Design review of the part built by this model. Coordinates are the model's own, in mm. A direction names the side the tool comes from. Coordinates: 2 decimals unless noted, no trailing zeros. Write each loop counter-clockwise with the first axis right and the second up, starting at its lowest first coordinate (ties: lowest second). Pieces come first, ordered by that corner, then holes. Notation, with made-up numbers: (-16.5, 12) - (36.5, 12) arc R26 ccw to (36.5, 37) - close; hole circle Ø1 at (-24, -22.75). An arc over 180 degrees is marked (long way). One line per item, written item: value.
from build123d import *

# Parameters (mm, degrees)
F0_R      = 38.1
F1_DEPTH  = 25.4
F2_W      = 25.4
F2_H      = 25.4
F3_DEPTH  = 25.4
F4_R      = 25.4
F5_DEPTH  = 25.4
F6_W      = 25.4
F6_H      = 25.4
F7_DEPTH  = 166
F8_W      = 25.4
F8_H      = 25.4
F9_DEPTH  = 76.201
F10_R     = 12.7
F11_DEPTH = 38.101
F12_DEPTH = 50.8
F13_W     = 25.4
F13_H     = 25.4
F14_DEPTH = 38.1010001
F15_W     = 25.4
F15_H     = 25.4
F16_DEPTH = 50.8010001


# Not quite as in the source:
# - an extrude ends at something that could not be found from the text; its depth is read off the source's solid


with BuildPart() as f1:
    # F0 (on Top) → F1 (new body)
    with BuildSketch(Plane.XY):
        Circle(F0_R)
    extrude(amount=F1_DEPTH)

    # F2 (on face) → F3 (join)
    with BuildSketch(Plane.XY.offset(25.4)):
        Rectangle(F2_W, F2_H)
    extrude(amount=F3_DEPTH)

    # F4 (on face) → F5 (join)
    with BuildSketch(Plane(origin=(0, 0, 0), x_dir=(1, 0, 0), z_dir=(0, 0, -1))):
        Circle(F4_R)
    extrude(amount=F5_DEPTH)

    # F6 (on face) → F7 (cut, through all)
    with BuildSketch(Plane(origin=(0, 0, -25.4), x_dir=(1, 0, 0), z_dir=(0, 0, -1))):
        Rectangle(F6_W, F6_H)
    extrude(amount=F7_DEPTH, mode=Mode.SUBTRACT)

    # F8 (on face) → F9 (cut, through all)
    with BuildSketch(Plane(origin=(0, 0, -25.4), x_dir=(1, 0, 0), z_dir=(0, 0, -1))):
        Rectangle(F8_W, F8_H)
    extrude(amount=-F9_DEPTH, mode=Mode.SUBTRACT)

    # F10 (on Front) → F11 (cut, through all)
    with BuildSketch(Plane.XZ):
        Circle(F10_R)
    extrude(amount=-F11_DEPTH, mode=Mode.SUBTRACT)

    # F10 (on Front) → F12 (cut)
    with BuildSketch(Plane.XZ):
        Circle(F10_R)
    extrude(amount=F12_DEPTH, mode=Mode.SUBTRACT)

    # F13 (on Right) → F14 (cut, through all)
    with BuildSketch(Plane.YZ):
        Rectangle(F13_W, F13_H)
    extrude(amount=-F14_DEPTH, mode=Mode.SUBTRACT)

    # F15 (on face) → F16 (cut, through all)
    with BuildSketch(Plane.YZ.offset(-12.7)):
        Rectangle(F15_W, F15_H)
    extrude(amount=F16_DEPTH, mode=Mode.SUBTRACT)


solid = f1.part
1. Consider section D-D, the plane z = 21.5. Write out the cut boundary in (x, y).
Answer block:
outline: circle Ø76.2 at (0, 0); hole (-12.7, -12.7) - (12.7, -12.7) - (12.7, 12.7) - (-12.7, 12.7) - close
2. Consider section C-C, the plane z = 8. Write out the cut boundary in (x, y).
Answer block:
outline: (-35.92, -12.7) arc R38.1 ccw to (-9.86, -36.8) - (-9.86, -12.7) - close; (-35.92, 12.7) - (-9.86, 12.7) - (-9.86, 36.8) arc R38.1 ccw to start; (9.86, -36.8) arc R38.1 ccw to (35.92, -12.7) - (9.86, -12.7) - close; (9.86, 12.7) - (35.92, 12.7) arc R38.1 ccw to (9.86, 36.8) - close
3. For faces 1 (the face through (-18.72, -17.17, -15.34)), 2 (the face through (-19, 0, -12.7)), 3 (the face through (-12.7, 0, -19)), list the 3-axis set-ups (+Z, -Z, +X, -X, +Y, -Y) from which the entire face can be reached by the end or side of a thin tool; tool diameter is ignored.
Answer block:
face 1: -Z
face 2: +X, -X
face 3: +Z, -Z
4. Mouldability with a two-part tool opening along Y and no side actions: class faces 4 (the face through (-25, 0, 12.7)), 5 (the face through (0, 17, -25.4)), 6 (the face through (17.58, -33.8, 15.34)) as released by +Y, released by -Y, zero draft, split by the parting line, or undercut.
Answer block:
face 4: undercut
face 5: zero draft
face 6: split by the parting line
5. Wall thickness on line 1 along Z through (x, y) = (0, -18.25); line 2 along Y through (x, z) = (-25, 6.5); line 3 along Y through (x, z) = (13.5, 5): over which ranges is each line inside the solid? List them lowest first.
Answer block:
line 1: z = -25.4 to -12.7, 12.7 to 25.4
line 2: y = -28.75 to -12.7, 12.7 to 28.75
line 3: y = -35.63 to -12.7, 12.7 to 35.63
6. Insertion check: pin 1 Ø8 at (x, z) = (-9, 5) entering from -Y; pin 2 Ø10 at (y, z) = (5.5, -16.5) entering from -X; pin 3 Ø11.5 at (x, y) = (-22, -22.5) entering from -Z. Each pin has a flat end and moves straight along its axis. Give the tip position at first contact, or say it passes through.
Answer block:
pin 1: stops at y = -37.03
pin 2: stops at x = -25.4
pin 3: stops at z = 0
7. Consider section A-A, the plane y = 0. Write out the cut boundary in (x, z), then the cut area to 3 significant figures.
Answer block:
outline: (-38.1, 12.7) - (-12.7, 12.7) - (-12.7, 25.4) - (-38.1, 25.4) - close; (-25.4, -25.4) - (-12.7, -25.4) - (-12.7, -12.7) - (-25.4, -12.7) - close; (12.7, -25.4) - (25.4, -25.4) - (25.4, -12.7) - (12.7, -12.7) - close; (12.7, 12.7) - (38.1, 12.7) - (38.1, 25.4) - (12.7, 25.4) - close
area: 968 mm^2
